Design review of the part built by this model. Coordinates are the model's own, in mm. A direction names the side the tool comes from. Give positions to 0.01 mm unless a question says otherwise; leave off trailing zeros. Order: outer loops, then holes, each group sorted by start corner. A loop starts at its lowest first (then second) coordinate and runs counter-clockwise, first axis right, second up. Notation, with made-up numbers: (89.25, 56) -> (112.25, 56) arc R22 cw to (112.25, 90) -> close; hole circle Ø6 at (80, -2). An arc over 180 degrees is marked (long way). One line per item, written item: value.
from build123d import *

# Parameters (mm, degrees)
F0_W     = 25.4
F0_H     = 25.4
F1_DEPTH = 25.4
F2_W     = 25.4
F2_H     = 25.4
F3_DEPTH = 25.4
F4_W     = 25.4
F4_H     = 25.4
F5_DEPTH = 25.4
F7_R     = 1.27
F6_R     = 1.27
F8_DEPTH = 25.4


with BuildPart() as f1:
    # F0 (on Front) → F1 (new body)
    with BuildSketch(Plane.XZ):
        Polygon((-50.8, 0), (-25.4, 0), (-25.4, 25.4), (-25.4, 50.8), (-50.8, 50.8), align=None)
        with Locations((-12.7, 12.7)):
            Rectangle(F0_W, F0_H)
    extrude(amount=F1_DEPTH)

    # F2 (on face) → F3 (join)
    with BuildSketch(Plane.XZ.offset(25.4)):
        with Locations((-12.7, 12.7)):
            Rectangle(F2_W, F2_H)
    extrude(amount=F3_DEPTH)

    # F4 (on face) → F5 (join)
    with BuildSketch(Plane(origin=(0, 0, 0), x_dir=(-1, 0, 0), z_dir=(0, 1, 0))):
        with Locations((12.7, 12.7)):
            Rectangle(F4_W, F4_H)
    extrude(amount=F5_DEPTH)

    # F7 (on face) + F6 (on face) → F8 (cut)
    with BuildSketch(Plane(origin=(-25.4, 0, 0), x_dir=(0, -1, 0), z_dir=(-1, 0, 0))):
        with Locations((38.1, 12.7)):
            Circle(F7_R)
    with BuildSketch(Plane(origin=(-25.4, 0, 0), x_dir=(0, -1, 0), z_dir=(-1, 0, 0))):
        with Locations((-12.7, 12.7)):
            Circle(F6_R)
    extrude(amount=-F8_DEPTH, mode=Mode.SUBTRACT)


solid = f1.part
Item 1: Draft analysis for pull direction Y (two halves, no side actions). For faces 6 (the flat face through (-13, -13, 25.4)), 7 (the cylindrical face through (-12.878, -37.164, 13.558)), 8 (the flat face through (-38, 0, 26)), state which applies: pulls with the +Y half, pulls with the -Y half, needs draft (parallel to the pull), parting line crosses it, or undercut.
Returned:
face 6: needs draft
face 7: undercut
face 8: pulls with the +Y half
Item 2: Add section A-A on y = 12.7. Give the boundary of the cut face in (x, z), plus the area to 3 significant figures.
Returned:
outline: (-25.4, 0) -> (0, 0) -> (0, 11.43) -> (-25.4, 11.43) -> close; (-25.4, 13.97) -> (0, 13.97) -> (0, 25.4) -> (-25.4, 25.4) -> close
area: 581 mm²
Item 3: Clearance check with flat-ended pins moving along their axes: P1, Ø20.5, axis at y = 12, z = 18, coming from the -X side; P2, Ø4, axis at x = -8, y = 12, coming from the +Z side; P3, Ø12.5, axis at x = -40, z = 35, coming from the -Y side. State where each tip first meets the part, or that it passes through.
Returned:
P1: x = -25.4
P2: z = 25.4
P3: y = -25.4
Item 4: Add section B-B on z = 12.7. Give the boundary of the cut face in (x, y).
Returned:
outline: (-50.8, -25.4) -> (-25.4, -25.4) -> (-25.4, -36.83) -> (0, -36.83) -> (0, 11.43) -> (-25.4, 11.43) -> (-25.4, 0) -> (-50.8, 0) -> close; (-25.4, -50.8) -> (0, -50.8) -> (0, -39.37) -> (-25.4, -39.37) -> close; (-25.4, 13.97) -> (0, 13.97) -> (0, 25.4) -> (-25.4, 25.4) -> close
Item 5: To check wall thickness, follow line 1 along Z through (x, y) = (-16.5, 12.7); line 2 along Z through (x, y) = (-19.5, 17); line 3 along Y through (x, z) = (-7, 12). State the ranges of each line that lie inside material, in increasing order. Write a range as from..to.
Returned:
line 1: 0..11.43, 13.97..25.4
line 2: 0..25.4
line 3: -50.8..-39.16, -37.04..11.64, 13.76..25.4
Item 6: Add section D-D on z = 22. Give the boundary of the cut face in (x, y).
Returned:
outline: (-50.8, -25.4) -> (-25.4, -25.4) -> (-25.4, -50.8) -> (0, -50.8) -> (0, 25.4) -> (-25.4, 25.4) -> (-25.4, 0) -> (-50.8, 0) -> close
Item 7: Add section C-C on x = -11. Give the boundary of the cut face in (y, z).
Returned:
outline: (-50.8, 0) -> (25.4, 0) -> (25.4, 25.4) -> (-50.8, 25.4) -> close; hole circle Ø2.54 at (-38.1, 12.7); hole circle Ø2.54 at (12.7, 12.7)
Item 8: Machinability: for faces 1 (the flat face through (-50.8, -13, 26)), 2 (the flat face through (-13, -50.8, 13)), 3 (the flat face through (-25.4, 13, 15)), 4 (the flat face through (-25.4, -13, 38)), 5 (the flat face through (-25.4, -38, 15)), which of the approach directions +Z, -Z, +X, -X, +Y, -Y give a long, thin tool a straight path to every point of the face, cutting with its end or side? Answer none if there is none.
Returned:
face 1: +Z, -Z, -X, +Y, -Y
face 2: +Z, -Z, +X, -X, -Y
face 3: +Z, -Z, -X, +Y
face 4: +Z, +X, +Y, -Y
face 5: +Z, -Z, -X, -Y
